Build history of the part. All positions in model axes, mm. Give positions to 0.01 mm unless a question says otherwise; leave off trailing zeros. Loops run counter-clockwise (first coordinate to the right, second up) from the corner with the lowest first, then second, coordinate; pieces in that order, holes last. Notation, with made-up numbers: (29.25, -28) -> (57.25, -28) arc R20 cw to (57.25, -19) -> close; hole circle Ø2 at (9.25, 34.25). An arc over 180 degrees is marked (long way). Answer in a Markdown table with one row per item. Add a question column.
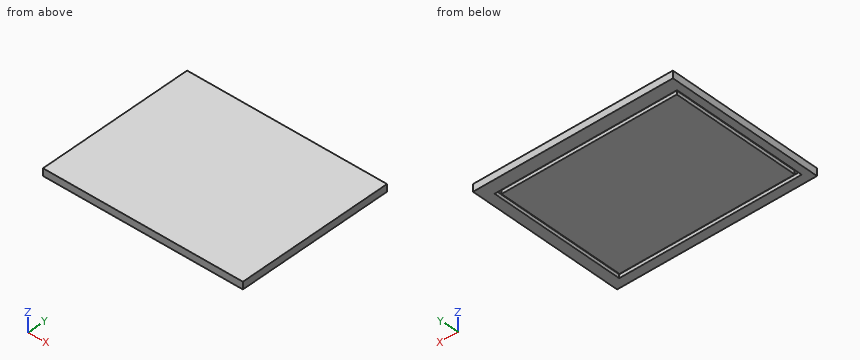
from build123d import *

# Parameters (mm, degrees)
SKETCH1_W           = 82.5
SKETCH1_H           = 65
BOSS_EXTRUDE1_DEPTH = 1.5
SKETCH2_W           = 75.322744119
SKETCH2_H           = 56.205881557
SKETCH2_W_2         = 72.322744119
SKETCH2_H_2         = 53.205881557
CUT_EXTRUDE1_DEPTH  = 1.5


with BuildPart() as part:
    # Sketch1 → Boss-Extrude1 (new, symmetric)
    with BuildSketch(Plane.XY):
        with Locations((0.253524641, 0.760573924)):
            Rectangle(SKETCH1_W, SKETCH1_H)
    extrude(amount=BOSS_EXTRUDE1_DEPTH, both=True)

    # Sketch2 → Cut-Extrude1 (cut)
    with BuildSketch(Plane(origin=(0, 0, -1.5), x_dir=(-1, 0, 0), z_dir=(0, 0, -1))):
        with Locations((0.340133491, -0.002700818)):
            Rectangle(SKETCH2_W, SKETCH2_H)
        with Locations((0.340133491, -0.002700818)):
            Rectangle(SKETCH2_W_2, SKETCH2_H_2, mode=Mode.SUBTRACT)
    extrude(amount=-CUT_EXTRUDE1_DEPTH, mode=Mode.SUBTRACT)


solid = part.part
(1) Saw through at B-B, the plane y = -14.5. List the corners of the cut face in (x, z).
(2) Saw through at A-A, the plane z = -0.65. List the corners of the cut face in (x, y).
(3) Saw through at C-C, the plane x = -15. List the corners of the cut face in (y, z), then the cut area to 4 significant figures.
(4) Wall check: line 1 along X through (y, z) = (-17.5, -0.7); line 2 along Y through (x, z) = (-16.5, -0.1). Give the ranges that are in metal, low to high. Write a range as from..to.
Worked answers:
| question | item | result |
|---|---|---|
| 1 | outline | (-41, -1.5) -> (-38, -1.5) -> (-38, 0) -> (-36.5, 0) -> (-36.5, -1.5) -> (35.82, -1.5) -> (35.82, 0) -> (37.32, 0) -> (37.32, -1.5) -> (41.5, -1.5) -> (41.5, 1.5) -> (-41, 1.5) -> close |
| 2 | outline | (-41, -31.74) -> (41.5, -31.74) -> (41.5, 33.26) -> (-41, 33.26) -> close; (-36.5, -26.61) -> (35.82, -26.61) -> (35.82, 26.6) -> (-36.5, 26.6) -> close; hole (-38, -28.11) -> (37.32, -28.11) -> (37.32, 28.1) -> (-38, 28.1) -> close |
| 3 | outline | (-31.74, -1.5) -> (-28.11, -1.5) -> (-28.11, 0) -> (-26.61, 0) -> (-26.61, -1.5) -> (26.6, -1.5) -> (26.6, 0) -> (28.1, 0) -> (28.1, -1.5) -> (33.26, -1.5) -> (33.26, 1.5) -> (-31.74, 1.5) -> close |
| 3 | area | 190.5 mm^2 |
| 4 | line 1 | -41..-38, -36.5..35.82, 37.32..41.5 |
| 4 | line 2 | -31.74..-28.11, -26.61..26.6, 28.1..33.26 |
